from build123d import *

# Parameters (mm, degrees)
SKETCH1_R                                           = 60.625
SKETCH1_R_2                                         = 45
BOSS_EXTRUDE1_DEPTH                                 = 4
SKETCH2_R                                           = 49
SKETCH2_R_2                                         = 45
BOSS_EXTRUDE2_DEPTH                                 = 52
SKETCH4_W                                           = 13.25
SKETCH4_H                                           = 8
SKETCH4_W_2                                         = 8
SKETCH4_H_2                                         = 38
BOSS_EXTRUDE4_DEPTH                                 = 13
BOSS_EXTRUDE5_DEPTH                                 = 4
SKETCH7_R                                           = 1.3
CUT_EXTRUDE4_DEPTH                                  = 7.2
SKETCH9_W                                           = 10
SKETCH9_H                                           = 24
CUT_EXTRUDE7_DEPTH                                  = 8
CUT_EXTRUDE9_DEPTH                                  = 101.273532151
CSK_FOR_M3_COUNTERSUNK_FLAT_HEAD_SCREW1_D           = 3.4
CSK_FOR_M3_COUNTERSUNK_FLAT_HEAD_SCREW1_CSINK_D     = 6.3
CSK_FOR_M3_COUNTERSUNK_FLAT_HEAD_SCREW1_CSINK_ANGLE = 90


with BuildPart() as part:
    # Sketch1 → Boss-Extrude1 (new body)
    with BuildSketch(Plane(origin=(0, 0, 0), x_dir=(1, 0, 0), z_dir=(0, 1, 0))):
        with Locations(Location((0, 0, 0), (0, 0, 270))):
            Circle(SKETCH1_R)
        with Locations(Location((0, 0, 0), (0, 0, 270))):
            Circle(SKETCH1_R_2, mode=Mode.SUBTRACT)
    extrude(amount=BOSS_EXTRUDE1_DEPTH)

    # Sketch2 → Boss-Extrude2 (add)
    with BuildSketch(Plane(origin=(0, 4, 0), x_dir=(1, 0, 0), z_dir=(0, 1, 0))):
        with Locations(Location((0, 0, 0), (0, 0, 90))):
            Circle(SKETCH2_R)
        with Locations(Location((0, 0, 0), (0, 0, 270))):
            Circle(SKETCH2_R_2, mode=Mode.SUBTRACT)
    extrude(amount=BOSS_EXTRUDE2_DEPTH)

    # Sketch4 → Boss-Extrude4 (add, symmetric)
    with BuildSketch(Plane.XY):
        with Locations((-38.375, 34)):
            Rectangle(SKETCH4_W, SKETCH4_H)
        Polygon((-31.75, 30), (-45, 30), (-45, 16.75), align=None)
        with Locations((15.25, 19)):
            Rectangle(SKETCH4_W_2, SKETCH4_H_2)
    extrude(amount=BOSS_EXTRUDE4_DEPTH, both=True)


with BuildPart() as boss_extrude4_piece_1:
    # of the separate pieces the step leaves, piece 1, a body of its own (boss_extrude4_pieces)
    add(part.part.solids().sort_by_distance((0, 0, 60.625))[0])



with BuildPart() as boss_extrude4_piece_2:
    # of the separate pieces the step leaves, piece 2, a body of its own (boss_extrude4_pieces)
    add(part.part.solids().sort_by_distance((11.25, 38, -13))[0])


with BuildPart() as boss_extrude4_piece_1_1:
    add(boss_extrude4_piece_1.part)

    add(boss_extrude4_piece_2.part)  # Boss-Extrude5 merges Boss-Extrude4 piece 2
    # Sketch5 → Boss-Extrude5 (add)
    with BuildSketch(Plane.XZ):
        with BuildLine():
            Line((11.25, 13), (29.067400866, 34.352382842))
            ThreePointArc((29.067400866, 34.352382842), (45, 0), (29.067400866, -34.352382842))
            Line((29.067400866, -34.352382842), (11.25, -13))
            Line((11.25, -13), (11.25, 13))
        make_face()
    extrude(amount=-BOSS_EXTRUDE5_DEPTH)

    # Sketch7 → Cut-Extrude4 (cut)
    with BuildSketch(Plane(origin=(0, 38, 0), x_dir=(1, 0, 0), z_dir=(0, 1, 0))):
        with Locations(Location((-34.25, 5, 0), (0, 0, 180))):
            Circle(SKETCH7_R)
        with Locations(Location((-34.25, -5, 0), (0, 0, 180))):
            Circle(SKETCH7_R)
        with Locations(Location((13.75, 5, 0), (0, 0, 180))):
            Circle(SKETCH7_R)
        with Locations(Location((13.75, -5, 0), (0, 0, 180))):
            Circle(SKETCH7_R)
    extrude(amount=-CUT_EXTRUDE4_DEPTH, mode=Mode.SUBTRACT)

    # Sketch9 → Cut-Extrude7 (cut)
    with BuildSketch(Plane.ZY.offset(-11.25)):
        with Locations((0, 17)):
            Rectangle(SKETCH9_W, SKETCH9_H)
    extrude(amount=-CUT_EXTRUDE7_DEPTH, mode=Mode.SUBTRACT)

    # Sketch12 → Cut-Extrude9 (cut, through all)
    with BuildSketch(Plane(origin=(0, 4, 0), x_dir=(1, 0, 0), z_dir=(0, 1, 0))):
        with BuildLine():
            Line((29.479537487, 22.359715328), (27.25, 19.687836398))
            Line((27.25, 19.687836398), (27.25, -19.687836398))
            Line((27.25, -19.687836398), (29.479537487, -22.359715328))
            ThreePointArc((29.479537487, -22.359715328), (37, 0), (29.479537487, 22.359715328))
        make_face()
        Polygon((27.25, -19.687836398), (27.25, 19.687836398), (24.25, 16.092634774), (24.25, -16.092634774), align=None)
    extrude(amount=-CUT_EXTRUDE9_DEPTH, mode=Mode.SUBTRACT)

    # CSK for M3 Countersunk Flat Head Screw1 (through all)
    with Locations(Plane(origin=(0, 4, 0), x_dir=(1, 0, 0), z_dir=(0, 1, 0))):
        with Locations((-38.890872965, 38.890872965), (-38.890872965, -38.890872965), (38.890872965, -38.890872965), (38.890872965, 38.890872965)):
            CounterSinkHole(CSK_FOR_M3_COUNTERSUNK_FLAT_HEAD_SCREW1_D / 2, CSK_FOR_M3_COUNTERSUNK_FLAT_HEAD_SCREW1_CSINK_D / 2, counter_sink_angle=CSK_FOR_M3_COUNTERSUNK_FLAT_HEAD_SCREW1_CSINK_ANGLE)


solid = boss_extrude4_piece_1_1.part
Geometry check sheet. Reference: the model listing, model coordinates, mm. A direction names the side the tool comes from. Round coordinates to 2 decimals unless told otherwise and drop trailing zeros. Order: outer loops, then holes, each group sorted by start corner. A loop starts at its lowest first (then second) coordinate and runs counter-clockwise, first axis right, second up. Notation, with made-up numbers: (-25, 55) - (18, 55) arc R32 cw to (18, 94) - close; hole circle Ø8 at (52.5, 14.5). An arc over 180 degrees is marked (long way). One line per question, with ' | ' between items. Start each with the question number.
(1) Depth check by flat-ended pin: pin 1 Ø9 at (x, y) = (15.5, 12.5) entering from +Z; pin 2 Ø3 at (x, y) = (-45.5, 45) entering from -Z; pin 3 Ø4 at (x, z) = (38.89, -38.89) entering from +Y; pin 4 Ø3 at (x, z) = (38.89, 38.89) entering from +Y. Enter the tip coordinate at first touch or a pass-through.
(2) Sectioned sample at B-B on y = 26.5. Record the cut outline in (x, z), and give its area (3 significant figures).
(3) Release check for a two-part mould opening along X. For faces 4 (the cylindrical face through (-36.9, 2, -48.1)), 5 (the flat face through (14, 0, 1)), 6 (the cylindrical face through (-40.46, 1.26, -38.24)) record: released by +X, released by -X, zero draft, split by the parting line, or undercut.
(4) Thickness scan on L1, parallel to X at y = 33.5, z = -6.5; L2, parallel to Z at x = -34, y = 36; L3, parallel to X at y = 35, z = 5.5. Record the ranges inside material, lowest first. Write a range as [from, to].
(5) Sectioned sample at D-D on y = 14. Record the cut outline in (x, z).
(6) Sectioned sample at C-C on z = 0. Record the cut outline in (x, y) (3 decimals).
(7) Sectioned sample at A-A on x = 0. Record the cut outline in (y, z) (3 decimals).
(8) Access from +Z, -Z, +X, -X, +Y, -Y to the whole of each face (thin tool, end or side, straight path). Record for faces 1 (the flat face through (-31.75, 34, 0)), 2 (the flat face through (15, 21, 13)), 3 (the flat face through (15, 29, 0)).
Conclusion:
1) pin 1: stops at z = 47.75 | pin 2: stops at z = -21.56 | pin 3: stops at y = 2.85 | pin 4: passes through
2) outline: circle Ø98 at (0, 0); (11.25, -13) - (19.25, -13) - (19.25, -5) - (11.25, -5) - close; (11.25, 5) - (19.25, 5) - (19.25, 13) - (11.25, 13) - close; hole (-43.08, -13) arc R45 ccw (long way) to (-43.08, 13) - (-35.25, 13) - (-35.25, -13) - close | area: 1,550 mm2
3) face 4: split by the parting line | face 5: zero draft | face 6: undercut
4) L1: x = [-48.57, -31.75], [11.25, 19.25], [44.53, 48.57] | L2: z = [-35.28, -29.48], [-13, -6.28], [-3.72, 3.72], [6.28, 13], [29.48, 35.28] | L3: x = [-48.69, -35.45], [-33.05, -31.75], [11.25, 12.55], [14.95, 19.25], [44.66, 48.69]
5) outline: circle Ø98 at (0, 0); (11.25, -13) - (19.25, -13) - (19.25, -5) - (11.25, -5) - close; (11.25, 5) - (19.25, 5) - (19.25, 13) - (11.25, 13) - close; hole circle Ø90 at (0, 0)
6) outline: (-60.625, 0) - (-45, 0) - (-45, 16.75) - (-31.75, 30) - (-31.75, 38) - (-45, 38) - (-45, 56) - (-49, 56) - (-49, 4) - (-60.625, 4) - close; (11.25, 0) - (24.25, 0) - (24.25, 4) - (19.25, 4) - (19.25, 5) - (11.25, 5) - close; (11.25, 29) - (19.25, 29) - (19.25, 38) - (11.25, 38) - close; (37, 0) - (60.625, 0) - (60.625, 4) - (49, 4) - (49, 56) - (45, 56) - (45, 4) - (37, 4) - close
7) outline: (0, -60.625) - (4, -60.625) - (4, -49) - (56, -49) - (56, -45) - (0, -45) - close; (0, 45) - (56, 45) - (56, 49) - (4, 49) - (4, 60.625) - (0, 60.625) - close
8) face 1: +Y, -Y | face 2: +Y | face 3: none
